Source: CAD feature listing. Evaluate the final solid. Frame: model axes, mm. Face numbers are marked on the shaded views. A direction names the side the tool comes from. Round coordinates to 2 decimals unless told otherwise and drop trailing zeros. Write each loop counter-clockwise with the first axis right and the second up, starting at its lowest first coordinate (ties: lowest second). Pieces come first, ordered by that corner, then holes. Notation, with made-up numbers: M -3.5,-37.5 L 27.5,-37.5 A21 ccw 27.5,-28.5 Z; hole C 61.25,-1.75 d4. An arc over 180 degrees is marked long. Use a Markdown table: item, result.
```python
from build123d import *

# Parameters (mm, degrees)
CUT_EXTRUDE1_DEPTH      = 1
CUT_EXTRUDE1_DEPTH_BACK = 6


with BuildPart() as part:
    # Sketch1 → Revolve1 (revolve)
    with BuildSketch(Plane.XY):
        Polygon((-20, 0), (-20, 6), (-12, 6), (-12, 5), (-10, 5), (-10, 8), (8, 8), (8, 10.5), (10, 12.5), (18, 12.5), (20, 10.5), (20, 0), align=None)
    revolve(axis=Axis((-20, 0, 0), (1, 0, 0)))

    # Sketch2 → Cut-Extrude1 (cut, two sides)
    with BuildSketch(Plane(origin=(20, 0, 0), x_dir=(0, 0, -1), z_dir=(1, 0, 0))) as cut_extrude1_sk:
        Polygon((0, 5.773502692), (-5, 2.886751346), (-5, -2.886751346), (0, -5.773502692), (5, -2.886751346), (5, 2.886751346), align=None)
    extrude(amount=CUT_EXTRUDE1_DEPTH, mode=Mode.SUBTRACT)
    extrude(cut_extrude1_sk.sketch, amount=-CUT_EXTRUDE1_DEPTH_BACK, mode=Mode.SUBTRACT)


solid = part.part
```
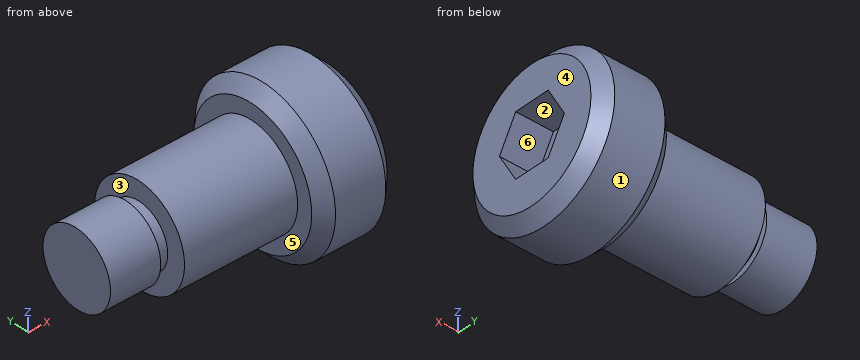
Q1. Section A-A on y = 0. Return loops of the section in (x, z), plus the area to 3 significant figures.
Results are:
| item | result |
|---|---|
| outline | M -20,-6 L -12,-6 L -12,-5 L -10,-5 L -10,-8 L 8,-8 L 8,-10.5 L 10,-12.5 L 18,-12.5 L 20,-10.5 L 20,-5 L 14,-5 L 14,5 L 20,5 L 20,10.5 L 18,12.5 L 10,12.5 L 8,10.5 L 8,8 L -10,8 L -10,5 L -12,5 L -12,6 L -20,6 Z |
| area | 636 mm^2 |
Q2. Line query: L1, parallel to X at y = 3, z = -4.25; L2, parallel to X at y = 8, z = 5.75; L3, parallel to X at y = 1.25, z = -7. Output: solid intervals per line, ascending.
Results are:
| item | result |
|---|---|
| L1 | -20 to -12, -10 to 14 |
| L2 | 8 to 20 |
| L3 | -10 to 20 |
Q3. Section B-B on x = -14. Return loops of the section in (y, z), plus the area to 3 significant figures.
Results are:
| item | result |
|---|---|
| outline | C 0,0 d12 |
| area | 113 mm^2 |
Q4. Reachability of the marked faces 4, 5 and 6 from +Z, -Z, +X, -X, +Y, -Y: full face, straight path, thin tool, end or side. Return the list, or none.
Results are:
| item | result |
|---|---|
| face 4 | +Z, -Z, +X, +Y, -Y |
| face 5 | -X |
| face 6 | +X |
Q5. First-contact query: pin 1 Ø6 at (x, y) = (5.5, 3) entering from +Z; pin 2 Ø4 at (x, z) = (1, 2) entering from -Y; pin 3 Ø5 at (x, y) = (-10, 9) entering from -Z. Flat tips, straight axial feed; report the tip coordinate or a pass-through.
Results are:
| item | result |
|---|---|
| pin 1 | z = 10.67 |
| pin 2 | y = -8 |
| pin 3 | z = -4.66 |
Q6. Mould query, pull axis Y, two halves, no side actions, for the marked faces 1, 2 and 3. Classes: +Y half, -Y half, draft (parallel to the pull), parting line (faces both ways), or undercut.
Results are:
| item | result |
|---|---|
| face 1 | parting line |
| face 2 | undercut |
| face 3 | draft |
Q7. Section C-C on x = -9.5. Return loops of the section in (y, z), plus the area to 3 significant figures.
Results are:
| item | result |
|---|---|
| outline | C 0,0 d16 |
| area | 201 mm^2 |
